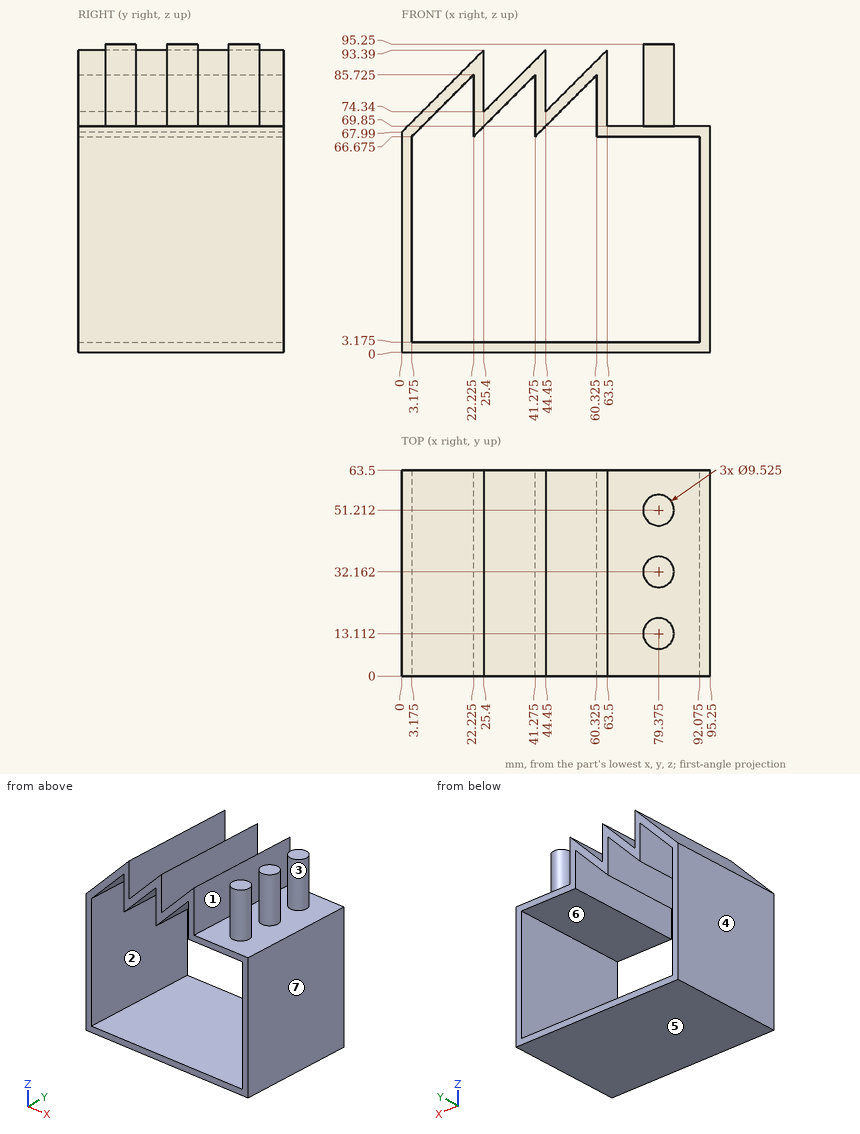
Print and shaded views of the part. All mm, measured from the part's lowest x, y and z. A direction names the side the tool comes from. Give positions to 0.01 mm unless a question says otherwise; leave off trailing zeros. One line per question, with ' | ' between items. Start each with the question number.
1) Probe L1, parallel to Z at x = 49.5, y = 13 (1 decimal); L2, parallel to Z at x = 60, y = 49 (1 decimal); L3, parallel to X at y = 43, z = 90. List the from-to ranges inside material, lowest first.
2) Pin check, flat tips, straight feed: pin 1 (21 mm diameter, centred on y = 38.5, z = 79, fed in from -X); pin 2 (21 mm diameter, centred on y = 45, z = 85.5, fed in from +X); pin 3 (4 mm diameter, centred on x = 72, y = 54.5, fed in from +Z). Stop position of each tip, or through.
3) 3-axis set-ups, long thin cutter, end or side, ignore diameter. For the marked faces 1, 2, 3 and 4: which of +Z, -Z, +X, -X, +Y, -Y reach the whole face in a straight line?
4) Two-plate mould, pull along X, no slides. Class the marked faces 5, 6 and 7: released by +X, released by -X, zero draft, split by the parting line, or undercut.
Return value:
1) L1: 0 to 3.2, 74.9 to 79.4 | L2: 0 to 3.2, 85.4 to 89.9 | L3: 22.01 to 25.4, 41.06 to 44.45, 60.11 to 63.5
2) pin 1: x = 0.51 | pin 2: x = 84.14 | pin 3: z = 69.85
3) face 1: +Z, +Y, -Y | face 2: +Y, -Y | face 3: +Z | face 4: +Z, -Z, -X, +Y, -Y
4) face 5: zero draft | face 6: undercut | face 7: released by +X
